```python
from build123d import *

# Parameters (mm, degrees)
SKETCH_1_R          = 27.5
SKETCH_1_R_2        = 13.5
EXTRUDE_1_DEPTH     = 2
SKETCH_2_R          = 1.525
CUT_EXTRUDE_1_DEPTH = 2
SKETCH_3_R          = 1.525
CUT_EXTRUDE_2_DEPTH = 2


with BuildPart() as part:
    # 草图1 → 凸台-拉伸1 (new body)
    with BuildSketch(Plane.XY):
        Circle(SKETCH_1_R)
        Circle(SKETCH_1_R_2, mode=Mode.SUBTRACT)
    extrude(amount=EXTRUDE_1_DEPTH)

    # 草图2 → 切除-拉伸1 (cut)
    with BuildSketch(Plane.XY.offset(2)):
        with Locations((0, 17.5)):
            Circle(SKETCH_2_R)
        with Locations((8.75, 15.155444566)):
            Circle(SKETCH_2_R)
        with Locations((15.155444566, 8.75)):
            Circle(SKETCH_2_R)
        with Locations((17.5, 0)):
            Circle(SKETCH_2_R)
        with Locations((15.155444566, -8.75)):
            Circle(SKETCH_2_R)
        with Locations((8.75, -15.155444566)):
            Circle(SKETCH_2_R)
        with Locations((0, -17.5)):
            Circle(SKETCH_2_R)
        with Locations((-8.75, -15.155444566)):
            Circle(SKETCH_2_R)
        with Locations((-15.155444566, -8.75)):
            Circle(SKETCH_2_R)
        with Locations((-17.5, 0)):
            Circle(SKETCH_2_R)
        with Locations((-15.155444566, 8.75)):
            Circle(SKETCH_2_R)
        with Locations((-8.75, 15.155444566)):
            Circle(SKETCH_2_R)
    extrude(amount=-CUT_EXTRUDE_1_DEPTH, mode=Mode.SUBTRACT)

    # 草图3 → 切除-拉伸2 (cut)
    with BuildSketch(Plane.XY.offset(2)):
        with Locations((0, 24.5)):
            Circle(SKETCH_3_R)
        with Locations((17.324116139, 17.324116139)):
            Circle(SKETCH_3_R)
        with Locations((24.5, 0)):
            Circle(SKETCH_3_R)
        with Locations((17.324116139, -17.324116139)):
            Circle(SKETCH_3_R)
        with Locations((0, -24.5)):
            Circle(SKETCH_3_R)
        with Locations((-17.324116139, -17.324116139)):
            Circle(SKETCH_3_R)
        with Locations((-24.5, 0)):
            Circle(SKETCH_3_R)
        with Locations((-17.324116139, 17.324116139)):
            Circle(SKETCH_3_R)
    extrude(amount=-CUT_EXTRUDE_2_DEPTH, mode=Mode.SUBTRACT)


solid = part.part
```
CAD build for the part. Positions are in the model's coordinates, mm. Coordinates: 2 decimals unless noted, no trailing zeros. Write each loop counter-clockwise with the first axis right and the second up, starting at its lowest first coordinate (ties: lowest second). Pieces come first, ordered by that corner, then holes. Notation, with made-up numbers: (-28, 0.5) -> (-16, 0.5) arc R22 cw to (-16, 38.5) -> close; hole circle Ø2 at (78, -34). An arc over 180 degrees is marked (long way). Return JSON: item names as keys, results as strings. Group by question number.
Q1. Cut at A-A, the plane x = 0. Give the cut face in (y, z) (3 decimals), then the cut area to 3 significant figures.
Q2. Cut at D-D, the plane z = 1.6. State how many separate pieces and enclosed holes the cut face has, then the cut area to 3 significant figures.
Q3. Drill centre lines: line 1 (Y direction, x = -14.5, z = 0.8); line 2 (Y direction, x = -18, z = 1.95); line 3 (Y direction, x = 17, z = 1.4). Where is each one in solid material? Low to high.
Q4. Cut at B-B, the plane y = -24.5. Give the cut face in (x, z) (3 decimals), then the cut area to 3 significant figures.
Q5. Pull direction Y, two halves, no side cores. Call faces 1 (the face through (-0.33, 16.01, 1.01)), 2 (the face through (-5.961, -26.846, 0.986)), 3 (the face through (-13, -6, 2)), 4 (the face through (-7.93, 16.44, 1.01)): released by +Y, released by -Y, zero draft, split by the parting line, or undercut.
Returned:
{
 "1": {"outline": "(-27.5, 0) -> (-26.025, 0) -> (-26.025, 2) -> (-27.5, 2) -> close; (-22.975, 0) -> (-19.025, 0) -> (-19.025, 2) -> (-22.975, 2) -> close; (-15.975, 0) -> (-13.5, 0) -> (-13.5, 2) -> (-15.975, 2) -> close; (13.5, 0) -> (15.975, 0) -> (15.975, 2) -> (13.5, 2) -> close; (19.025, 0) -> (22.975, 0) -> (22.975, 2) -> (19.025, 2) -> close; (26.025, 0) -> (27.5, 0) -> (27.5, 2) -> (26.025, 2) -> close", "area": "31.6 mm2"},
 "2": {"separate pieces": "1", "enclosed holes": "21", "area": "1,660 mm2"},
 "3": {"line 1": "y = -23.37 to -10.13, -7.37 to 7.37, 10.13 to 23.37", "line 2": "y = -20.79 to -18.69, -15.96 to -1.44, 1.44 to 15.96, 18.69 to 20.79", "line 3": "y = -21.62 to -18.81, -15.83 to -1.44, 1.44 to 15.83, 18.81 to 21.62"},
 "4": {"outline": "(-12.49, 0) -> (-1.525, 0) -> (-1.525, 2) -> (-12.49, 2) -> close; (1.525, 0) -> (12.49, 0) -> (12.49, 2) -> (1.525, 2) -> close", "area": "43.9 mm2"},
 "5": {"face 1": "undercut", "face 2": "split by the parting line", "face 3": "zero draft", "face 4": "undercut"}
}
